Model file for the job. Use its own axes, mm. Give positions to 0.01 mm unless a question says otherwise; leave off trailing zeros. Loops run counter-clockwise (first coordinate to the right, second up) from the corner with the lowest first, then second, coordinate; pieces in that order, holes last. Notation, with made-up numbers: M 27.5,61.5 L 74.5,61.5 A37 cw 74.5,99.5 Z; hole C -9.75,6 d4. An arc over 180 degrees is marked long. Use CSV: the item, a comma, the result in double quotes. Start each with the question number.
(1) Slice it at C-C on y = 244.5. List the corners of the cut face in (x, z), and give its area (3 significant figures).
(2) Wall check: line 1 along X through (y, z) = (232.5, 453.8); line 2 along X through (y, z) = (228.5, 456); line 3 along Y through (x, z) = (248, 456). Give the ranges that are in metal, low to high. Write a range as from..to.
(3) Flat gauge pins, fed straight in: P1, Ø4, axis at x = 248, y = 228.5, coming from the -Z side; P2, Ø2, axis at x = 243, z = 453.8, coming from the +Y side. Where does each tip first touch, or does it go through?
(4) Slice it at D-D on x = 243. List the corners of the cut face in (y, z).
(5) Slice it at A-A on y = 228.5. List the corners of the cut face in (x, z), and give its area (3 significant figures).
(6) Slice it at B-B on z = 450.5. List the corners of the cut face in (x, y), and give its area (3 significant figures).
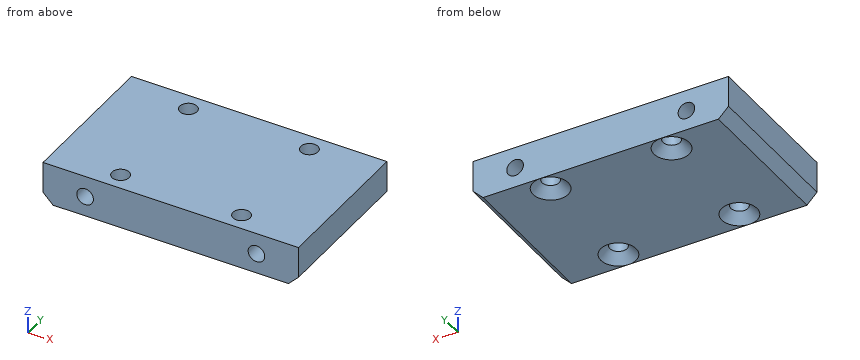
```python
from build123d import *

# Parameters (mm, degrees)
SKETCH_1_W                  = 50.700001454
SKETCH_1_H                  = 30.000001519
EXTRUDE_1_DEPTH             = 8.20000004
HOLE_WIZARD_3_3_3_3_1_D     = 3.300000535
HOLE_WIZARD_3_3_3_3_1_DEPTH = 30.00000152
HOLE_WIZARD_3_4_3_4_1_D     = 3.4
HOLE_WIZARD_3_4_3_4_1_DEPTH = 8.20000004
HOLE_WIZARD_3_4_3_4_2_D     = 3.4
HOLE_WIZARD_3_4_3_4_2_DEPTH = 8.20000004
CHAMFER_1_SIZE              = 1.8
CHAMFER_2_SIZE2             = 2.000000328
CHAMFER_2_SIZE              = 2.000000095


with BuildPart() as part:
    # 草图1 → 凸台-拉伸1 (new body)
    with BuildSketch(Plane(origin=(0, 0, 449.800000759), x_dir=(-1, 0, 0), z_dir=(0, 0, -1))):
        with Locations((-260.000000326, 239.999999943)):
            Rectangle(SKETCH_1_W, SKETCH_1_H)
    extrude(amount=-EXTRUDE_1_DEPTH)

    # Ø3.3 (3.3) 直径孔1
    with Locations(Plane(origin=(0, 224.999999183, 0), x_dir=(-1, 0, 0), z_dir=(0, -1, 0))):
        with Locations((-277.000001292, -453.79999995), (-243.000000389, -453.799999743)):
            Hole(HOLE_WIZARD_3_3_3_3_1_D / 2, depth=HOLE_WIZARD_3_3_3_3_1_DEPTH)

    # Ø3.4 (3.4) 直径孔1
    with Locations(Plane(origin=(0, 0, 449.800000759), x_dir=(-1, 0, 0), z_dir=(0, 0, -1))):
        with Locations((-272, 251.5), (-272, 228.5)):
            Hole(HOLE_WIZARD_3_4_3_4_1_D / 2, depth=HOLE_WIZARD_3_4_3_4_1_DEPTH)

    # Ø3.4 (3.4) 直径孔2
    with Locations(Plane.XY.offset(458.0000008)):
        with Locations((248, 251.5), (248, 228.5)):
            Hole(HOLE_WIZARD_3_4_3_4_2_D / 2, depth=HOLE_WIZARD_3_4_3_4_2_DEPTH)

    # 倒角1
    chamfer_1_edges = [part.edges().sort_by_distance(p)[0] for p in [
        (270.3, 228.5, 449.800000759),
        (270.3, 251.5, 449.800000759),
        (249.7, 228.5, 449.80000076),
        (249.7, 251.5, 449.80000076),
    ]]
    chamfer(chamfer_1_edges, length=CHAMFER_1_SIZE)

    # 倒角2
    chamfer_2_edges = [part.edges().sort_by_distance(p)[0] for p in [
        (234.649999599, 239.999999942, 449.800000759),
        (285.350001053, 239.999999942, 449.800000759),
    ]]
    chamfer(chamfer_2_edges, length=CHAMFER_2_SIZE, length2=CHAMFER_2_SIZE2)


solid = part.part
```
Reply:
1,outline,"M 234.65,451.8 L 236.65,449.8 L 283.35,449.8 L 285.35,451.8 L 285.35,458 L 234.65,458 Z; hole C 243,453.8 d3.3; hole C 277,453.8 d3.3"
1,area,"395 mm^2"
2,line 1,"x = 234.65..241.35, 244.65..275.35, 278.65..285.35"
2,line 2,"x = 234.65..246.3, 249.7..270.3, 273.7..285.35"
2,line 3,"y = 225..226.8, 230.2..249.8, 253.2..255"
3,P1,"stops at z = 451.3"
3,P2,"passes through"
4,outline,"M 225,449.8 L 255,449.8 L 255,452.15 L 225,452.15 Z; M 225,455.45 L 255,455.45 L 255,458 L 225,458 Z"
5,outline,"M 234.65,451.8 L 236.65,449.8 L 244.5,449.8 L 246.3,451.6 L 246.3,458 L 234.65,458 Z; M 249.7,451.6 L 251.5,449.8 L 268.5,449.8 L 270.3,451.6 L 270.3,458 L 249.7,458 Z; M 273.7,451.6 L 275.5,449.8 L 283.35,449.8 L 285.35,451.8 L 285.35,458 L 273.7,458 Z; hole C 243,453.8 d3.3; hole C 277,453.8 d3.3"
5,area,"332 mm^2"
6,outline,"M 235.95,225 L 284.05,225 L 284.05,255 L 235.95,255 Z; hole C 248,228.5 d5.6; hole C 248,251.5 d5.6; hole C 272,228.5 d5.6; hole C 272,251.5 d5.6"
6,area,"1,340 mm^2"
